The drawing under review shows one solid part. Ordinate dimensions are in mm from its lowest x, y, z. Give positions to 0.01 mm unless a question says otherwise; leave off trailing zeros. Order: outer loops, then holes, each group sorted by start corner. A loop starts at its lowest first (then second) coordinate and runs counter-clockwise, first axis right, second up. Notation, with made-up numbers: (41.25, 83) -> (54.25, 83) arc R30 cw to (54.25, 122) -> close; hole circle Ø1 at (1, 57.5). An arc over 180 degrees is marked (long way). One line per item, written item: value.
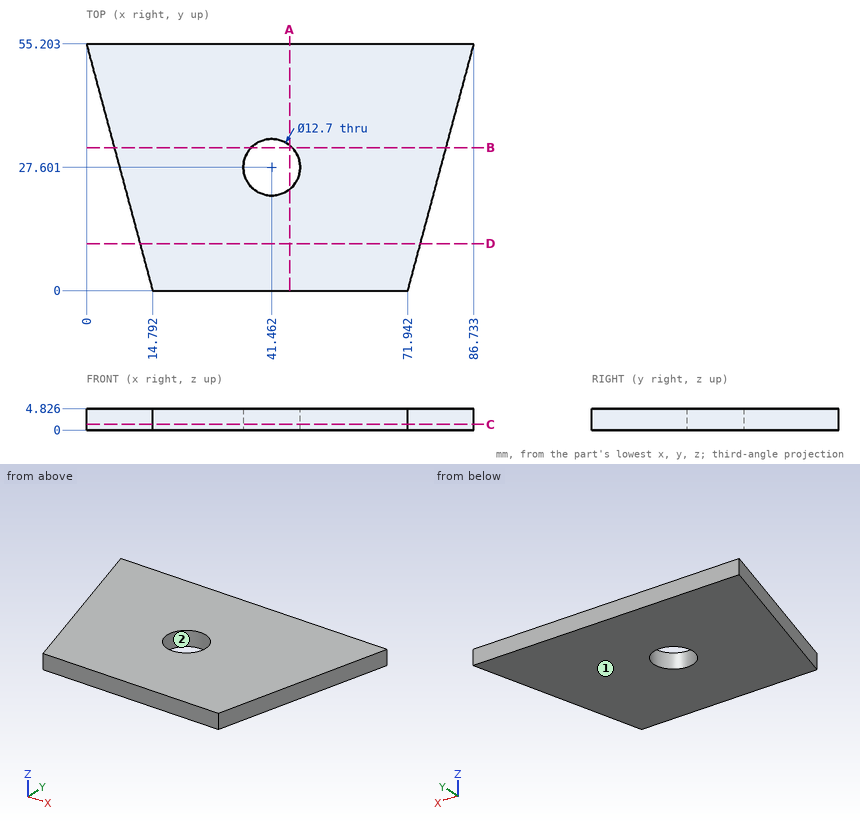
Item 1: Add section A-A on x = 45.5. Give the boundary of the cut face in (y, z), plus the area to 3 significant figures.
Returned:
outline: (0, 0) -> (22.7, 0) -> (22.7, 4.83) -> (0, 4.83) -> close; (32.5, 0) -> (55.2, 0) -> (55.2, 4.83) -> (32.5, 4.83) -> close
area: 219 mm²
Item 2: Add section D-D on y = 10.5. Give the boundary of the cut face in (x, z) (1 decimal).
Returned:
outline: (12, 0) -> (74.8, 0) -> (74.8, 4.8) -> (12, 4.8) -> close
Item 3: Add section B-B on y = 32. Give the boundary of the cut face in (x, z) (1 decimal).
Returned:
outline: (6.2, 0) -> (36.9, 0) -> (36.9, 4.8) -> (6.2, 4.8) -> close; (46, 0) -> (80.5, 0) -> (80.5, 4.8) -> (46, 4.8) -> close
Item 4: To check wall thickness, follow line 1 along Y through (x, z) = (47, 1.3) (1 decimal); line 2 along X through (y, z) = (25.5, 1.65) (1 decimal); line 3 along Y through (x, z) = (38, 0.8) (1 decimal). State the ranges of each line that lie inside material, in increasing order. Write a range as from..to.
Returned:
line 1: 0..24.5, 30.7..55.2
line 2: 8..35.5, 47.5..78.8
line 3: 0..22.3, 32.9..55.2
Item 5: Draft analysis for pull direction Y (two halves, no side actions). For the marked faces 1 and 2, state which applies: pulls with the +Y half, pulls with the -Y half, needs draft (parallel to the pull), parting line crosses it, or undercut.
Returned:
face 1: needs draft
face 2: undercut
Item 6: Add section C-C on z = 1.3. Give the boundary of the cut face in (x, y).
Returned:
outline: (0, 55.2) -> (14.79, 0) -> (71.94, 0) -> (86.73, 55.2) -> close; hole circle Ø12.7 at (41.46, 27.6)
